Verification items for the finished model (mm, model axes). A direction names the side the tool comes from. Coordinates: 2 decimals unless noted, no trailing zeros. Loops run counter-clockwise (first coordinate to the right, second up) from the corner with the lowest first, then second, coordinate; pieces in that order, holes last.
Q1. Mould release check, pull along X, two halves, no side actions. Record for faces 4 (the face through (-62.3, -20.7, 10.8)), 5 (the face through (0, -64, 22)), 6 (the face through (34.391, -65.153, 10.846)): +X half, -X half, draft (parallel to the pull), parting line (faces both ways), or undercut.
Q2. Sectioned sample at D-D (y = -30.5). Enter the section's corners in (x, z), then the cut area to 3 significant figures.
Q3. Sectioned sample at B-B (z = 15.25). Enter the section's corners in (x, y).
Q4. Material ranges on probe 1 along X at (y, z) = (-27, 12.5); probe 2 along Y at (x, z) = (57.5, 3.5); probe 3 along X at (y, z) = (-60, 1.5), recorded low to high.
Q5. Access from +Z, -Z, +X, -X, +Y, -Y to the whole of each face (thin tool, end or side, straight path). Record for faces 1 (the face through (52.687, -30.588, 10.846)), 2 (the face through (76.62, -10.66, 10.85)), 3 (the face through (-61.807, -29.486, 10.846)).
Q6. Go/stop test with flat-tipped pins: P1, Ø10, axis at x = -30.5, z = 10.5, coming from the -Y side; P2, Ø5.5, axis at x = 56.83, y = -25.03, coming from the +Z side; P3, Ø10, axis at x = -62.5, z = 4, coming from the -Y side; P4, Ø5, axis at y = -40.5, z = 6.5, coming from the +X side. Record where each tip stops, or that it passes through.
Q7. Sectioned sample at C-C (x = 5.5). Enter the section's corners in (y, z), then the cut area to 3 significant figures.
Q8. Sectioned sample at A-A (y = -17). Enter the section's corners in (x, z), then the cut area to 3 significant figures.
```python
from build123d import *

# Parameters (mm, degrees)
ESBO_O1_R                = 3
RESSALTO_EXTRUS_O1_DEPTH = 22


with BuildPart() as part:
    # Esboço1 → Ressalto-extrusão1 (new body)
    with BuildSketch(Plane.XY):
        with BuildLine():
            Line((-88.131389681, -3.713128135), (-88.131389681, -9.332118261))
            ThreePointArc((-88.131389681, -9.332118261), (-61.477752384, -29.824983348), (-41.890064111, -57.150728877))
            ThreePointArc((-41.890064111, -57.150728877), (-34.522230169, -65.073584532), (-24.106246719, -68))
            Line((-24.106246719, -68), (24.106246719, -68))
            ThreePointArc((24.106246719, -68), (34.522230169, -65.073584532), (41.890064111, -57.150728877))
            ThreePointArc((41.890064111, -57.150728877), (61.477752384, -29.824983348), (88.131389681, -9.332118261))
            Line((88.131389681, -9.332118261), (88.131389681, -3.713128135))
            ThreePointArc((88.131389681, -3.713128135), (76.464485554, -10.766043703), (65.672853174, -19.096766389))
            ThreePointArc((65.672853174, -19.096766389), (62.313137169, -20.69951591), (58.606836852, -20.353343104))
            ThreePointArc((58.606836852, -20.353343104), (53.244280911, -21.549279065), (52.217380785, -26.94675488))
            ThreePointArc((52.217380785, -26.94675488), (52.679803055, -30.640352489), (51.183377998, -34.048755298))
            ThreePointArc((51.183377998, -34.048755298), (50.828817615, -34.48677936), (50.476318173, -34.926463665))
            ThreePointArc((50.476318173, -34.926463665), (43.531544854, -44.57485582), (37.575499443, -54.863046658))
            ThreePointArc((37.575499443, -54.863046658), (32.049623987, -60.805188399), (24.2376364, -63))
            Line((24.2376364, -63), (-24.2376364, -63))
            ThreePointArc((-24.2376364, -63), (-32.049623987, -60.805188399), (-37.575499443, -54.863046658))
            ThreePointArc((-37.575499443, -54.863046658), (-43.531544854, -44.57485582), (-50.476318173, -34.926463665))
            ThreePointArc((-50.476318173, -34.926463665), (-50.828817615, -34.48677936), (-51.183377998, -34.048755298))
            ThreePointArc((-51.183377998, -34.048755298), (-52.679803055, -30.640352489), (-52.217380785, -26.94675488))
            ThreePointArc((-52.217380785, -26.94675488), (-53.244280911, -21.549279065), (-58.606836852, -20.353343104))
            ThreePointArc((-58.606836852, -20.353343104), (-62.313137169, -20.69951591), (-65.672853174, -19.096766389))
            ThreePointArc((-65.672853174, -19.096766389), (-76.464485554, -10.766043703), (-88.131389681, -3.713128135))
        make_face()
        with Locations((-56.834913612, -25.028841797)):
            Circle(ESBO_O1_R, mode=Mode.SUBTRACT)
        with Locations((56.834913612, -25.028841797)):
            Circle(ESBO_O1_R, mode=Mode.SUBTRACT)
    extrude(amount=RESSALTO_EXTRUS_O1_DEPTH)


solid = part.part
```
Geometry check:
1. face 4: undercut
1. face 5: draft
1. face 6: +X half
2. outline: (-60.83, 0) - (-52.7, 0) - (-52.7, 22) - (-60.83, 22) - close; (52.7, 0) - (60.83, 0) - (60.83, 22) - (52.7, 22) - close
2. area: 358 mm2
3. outline: (-88.13, -9.33) arc R115 cw to (-41.89, -57.15) arc R20 ccw to (-24.11, -68) - (24.11, -68) arc R20 ccw to (41.89, -57.15) arc R115 cw to (88.13, -9.33) - (88.13, -3.71) arc R120 ccw to (65.67, -19.1) arc R7 cw to (58.61, -20.35) arc R5 ccw to (52.22, -26.95) arc R7 cw to (51.18, -34.05) arc R120 ccw to (50.48, -34.93) arc R120 ccw to (37.58, -54.86) arc R15 cw to (24.24, -63) - (-24.24, -63) arc R15 cw to (-37.58, -54.86) arc R120 ccw to (-50.48, -34.93) arc R120 ccw to (-51.18, -34.05) arc R7 cw to (-52.22, -26.95) arc R5 ccw to (-58.61, -20.35) arc R7 cw to (-65.67, -19.1) arc R120 ccw to (-88.13, -3.71) - close; hole circle Ø6 at (-56.83, -25.03); hole circle Ø6 at (56.83, -25.03)
4. probe 1: x = -64.31 to -59.1, -54.57 to -52.24, 52.24 to 54.57, 59.1 to 64.31
4. probe 2: y = -34.15 to -27.95, -22.1 to -20.07
4. probe 3: x = -40.11 to -33.24, 33.24 to 40.11
5. face 1: +Z, -Z
5. face 2: +Z, -Z, +Y
5. face 3: +Z, -Z, -X, -Y
6. P1: stops at y = -67.95
6. P2: passes through
6. P3: stops at y = -34.15
6. P4: stops at x = 54.29
7. outline: (-68, 0) - (-63, 0) - (-63, 22) - (-68, 22) - close
7. area: 110 mm2
8. outline: (-76.18, 0) - (-68.16, 0) - (-68.16, 22) - (-76.18, 22) - close; (68.16, 0) - (76.18, 0) - (76.18, 22) - (68.16, 22) - close
8. area: 353 mm2
